```python
from build123d import *

# Parameters (mm, degrees)
SKETCH_1_W          = 42
SKETCH_1_H          = 42
EXTRUDE_1_DEPTH     = 40
SKETCH_2_R          = 11
EXTRUDE_2_DEPTH     = 2
SKETCH_3_R          = 1.5
CUT_EXTRUDE_1_DEPTH = 40
SKETCH_4_R          = 2.5
EXTRUDE_3_DEPTH     = 22
CUT_EXTRUDE_START   = -18
CUT_EXTRUDE_2_DEPTH = 18


with BuildPart() as part:
    # 草图1 → 凸台-拉伸1 (new body)
    with BuildSketch(Plane(origin=(0, 0, 0), x_dir=(1, 0, 0), z_dir=(0, 1, 0))):
        with Locations((21, 21)):
            Rectangle(SKETCH_1_W, SKETCH_1_H)
    extrude(amount=EXTRUDE_1_DEPTH)

    # 草图2 → 凸台-拉伸2 (add)
    with BuildSketch(Plane(origin=(0, 40, 0), x_dir=(1, 0, 0), z_dir=(0, 1, 0))):
        with Locations(Location((21, 21, 0), (0, 0, 270))):
            Circle(SKETCH_2_R)
    extrude(amount=EXTRUDE_2_DEPTH)

    # 草图3 → 切除-拉伸1 (cut)
    with BuildSketch(Plane.XZ):
        with Locations(Location((5.5, -36.5, 0), (0, 0, 270))):
            Circle(SKETCH_3_R)
        with Locations(Location((36.5, -36.5, 0), (0, 0, 270))):
            Circle(SKETCH_3_R)
        with Locations(Location((36.5, -5.5, 0), (0, 0, 270))):
            Circle(SKETCH_3_R)
        with Locations(Location((5.5, -5.5, 0), (0, 0, 270))):
            Circle(SKETCH_3_R)
    extrude(amount=-CUT_EXTRUDE_1_DEPTH, mode=Mode.SUBTRACT)

    # 草图4 → 凸台-拉伸3 (add)
    with BuildSketch(Plane(origin=(0, 42, 0), x_dir=(1, 0, 0), z_dir=(0, 1, 0))):
        with Locations(Location((21, 21, 0), (0, 0, 270))):
            Circle(SKETCH_4_R)
    extrude(amount=EXTRUDE_3_DEPTH)

    # 草图6 → 切除-拉伸2 (cut)
    with BuildSketch(Plane(origin=(0, 64, 0), x_dir=(1, 0, 0), z_dir=(0, 1, 0)).offset(CUT_EXTRUDE_START)):
        with BuildLine():
            Line((22.5, 23), (22.5, 21))
            Line((22.5, 21), (22.5, 19))
            ThreePointArc((22.5, 19), (23.236067977, 19.881966011), (23.5, 21))
            ThreePointArc((23.5, 21), (23.236067977, 22.118033989), (22.5, 23))
        make_face()
    extrude(amount=CUT_EXTRUDE_2_DEPTH, mode=Mode.SUBTRACT)


solid = part.part
```
Work out the finished part from the listing and answer in its coordinate system (mm). A direction names the side the tool comes from. Coordinates: 2 decimals unless noted, no trailing zeros. Loops run counter-clockwise (first coordinate to the right, second up) from the corner with the lowest first, then second, coordinate; pieces in that order, holes last. Notation, with made-up numbers: (81, -35.5) - (95, -35.5) arc R24 cw to (95, -13.5) - close; hole circle Ø4 at (77.25, 59.25). An arc over 180 degrees is marked (long way). Use a Markdown table: item, result.
Item 1: Find section C-C, the plane y = 38.5. Determine the outline of the cut face in (x, z).
Evaluation:
| item | result |
|---|---|
| outline | (0, -42) - (42, -42) - (42, 0) - (0, 0) - close; hole circle Ø3 at (5.5, -36.5); hole circle Ø3 at (5.5, -5.5); hole circle Ø3 at (36.5, -36.5); hole circle Ø3 at (36.5, -5.5) |
Item 2: For faces 1 (the flat face through (21, 64, -21)), 2 (the flat face through (30, 40, -12)), 3 (the flat face through (22.5, 55, -21)), determine the directions among +Z, -Z, +X, -X, +Y, -Y from which every point of the face is accessible in a straight line to the end or side of a thin tool.
Evaluation:
| item | result |
|---|---|
| face 1 | +Z, -Z, +X, -X, +Y |
| face 2 | +Y |
| face 3 | +Z, -Z, +X, +Y |
Item 3: The mould has two halves that part along X. Classify faces 4 (the cylindrical face through (4.6, 19.7, -35.3)), 5 (the cylindrical face through (5.57, 19.72, -4)), 6 (the flat face through (42, 20, -21)), 7 (the cylindrical face through (18.56, 52.85, -21.54)): +X half, -X half, draft (parallel to the pull), parting line (faces both ways), or undercut.
Evaluation:
| item | result |
|---|---|
| face 4 | undercut |
| face 5 | undercut |
| face 6 | +X half |
| face 7 | parting line |
Item 4: Consider probe 1 along X at (y, z) = (14, -36.5); probe 2 along X at (y, z) = (32, -36); probe 3 along Z at (x, y) = (5, 24). Determine where each line is inside the solid, lowest interval first. Write a range as from..to.
Evaluation:
| item | result |
|---|---|
| probe 1 | x = 0..4, 7..35, 38..42 |
| probe 2 | x = 0..4.09, 6.91..35.09, 37.91..42 |
| probe 3 | z = -42..-37.91, -35.09..-6.91, -4.09..0 |
Item 5: Find section B-B, the plane z = -5.5. Determine the outline of the cut face in (x, y).
Evaluation:
| item | result |
|---|---|
| outline | (0, 0) - (4, 0) - (4, 40) - (0, 40) - close; (7, 0) - (35, 0) - (35, 40) - (7, 40) - close; (38, 0) - (42, 0) - (42, 40) - (38, 40) - close |
Item 6: Given pin 1 Ø5 at (x, z) = (5.5, -5.5) entering from +Y; pin 2 Ø2 at (y, z) = (52, -20) entering from +X; pin 3 Ø0.8 at (x, z) = (23, -20.5) entering from +Y, each flat-ended and moving along its own axis, determine where each tip first touches the part or whether it passes through.
Evaluation:
| item | result |
|---|---|
| pin 1 | stops at y = 40 |
| pin 2 | stops at x = 22.5 |
| pin 3 | stops at y = 46 |
Item 7: Find section A-A, the plane x = 5.5. Determine the outline of the cut face in (y, z), and give its area (3 significant figures).
Evaluation:
| item | result |
|---|---|
| outline | (0, -42) - (40, -42) - (40, -38) - (0, -38) - close; (0, -35) - (40, -35) - (40, -7) - (0, -7) - close; (0, -4) - (40, -4) - (40, 0) - (0, 0) - close |
| area | 1,440 mm2 |
Item 8: Find section D-D, the plane z = -21. Determine the outline of the cut face in (x, y).
Evaluation:
| item | result |
|---|---|
| outline | (0, 0) - (42, 0) - (42, 40) - (32, 40) - (32, 42) - (23.5, 42) - (23.5, 46) - (22.5, 46) - (22.5, 64) - (18.5, 64) - (18.5, 42) - (10, 42) - (10, 40) - (0, 40) - close |
